For this review, take the finished solid that the model builds, in its own axes (mm). Round coordinates to 2 decimals unless told otherwise and drop trailing zeros. Write each loop counter-clockwise with the first axis right and the second up, starting at its lowest first coordinate (ties: lowest second). Pieces come first, ordered by that corner, then holes. Notation, with made-up numbers: (46, 86.5) -> (51, 86.5) arc R33 ccw to (51, 114.5) -> close; hole circle Ø1 at (71, 6). An arc over 180 degrees is marked (long way). Answer as CSV lines item,"result". Start each with the question number.
Item 1: Take a section at B-B on x = -5.5. Give the boundary of the cut face in (y, z).
Item 2: Wall thickness on probe 1 along Z at (x, y) = (4.5, -0.1); probe 2 along X at (y, z) = (-1.3, 112); probe 3 along Z at (x, y) = (3, -0.9): over which ranges is each line inside the solid? List them lowest first. Write a range as from..to.
Item 3: For pin 1 Ø1.5 at (y, z) = (-1.5, 98.5) entering from +X, flat-tipped, find the tip position at first contact; note if it passes through.
Item 4: Take a section at C-C on z = 44.5. Give the boundary of the cut face in (x, y), then the cut area to 3 significant figures.
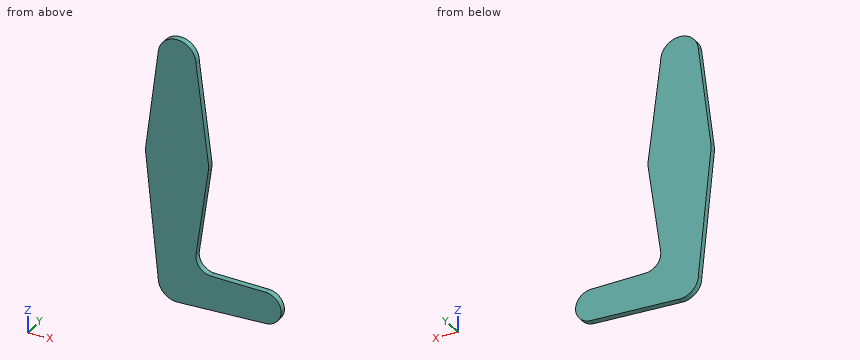
```python
from build123d import *

# Parameters (mm, degrees)
F0_R     = 3.175
F1_DEPTH = 3.048


with BuildPart() as f1:
    # F0 (on Front) → F1 (new body)
    with BuildSketch(Plane.XZ):
        with BuildLine():
            ThreePointArc((9.525, 114.3), (0.596483242, 123.8063048942), (-9.4502929642, 115.490625))
            ThreePointArc((-9.4502929642, 115.490625), (-7.14375, 107.9998046905), (0, 104.775))
            ThreePointArc((0, 104.775), (6.7351920908, 107.5648079092), (9.525, 114.3))
        make_face()
        with BuildLine():
            ThreePointArc((3.175, 114.3), (2.2450640303, 112.0549359697), (0, 111.125))
            ThreePointArc((0, 111.125), (-2.2450640303, 116.5450640303), (3.175, 114.3))
        make_face(mode=Mode.SUBTRACT)
        with BuildLine():
            Line((0, 47.625), (0, 9.525))
            ThreePointArc((0, 9.525), (6.7351920908, 6.7351920908), (9.525, 0))
            Line((9.525, 0), (36.5125, 0))
            ThreePointArc((36.5125, 0), (38.8886909991, 5.663545572), (44.5945783487, 7.9361831727))
            Line((44.5945783487, 7.9361831727), (17.2606145929, 8.4341428668))
            ThreePointArc((17.2606145929, 8.4341428668), (11.3562252192, 11.224257518), (9.5333913565, 17.4951290964))
            Line((9.5333913565, 17.4951290964), (15.7189155447, 61.2793426425))
            ThreePointArc((15.7189155447, 61.2793426425), (10.4106361345, 51.5152480094), (0, 47.625))
        make_face()
        with BuildLine():
            ThreePointArc((-15.7942028036, 61.9003804205), (-10.644756084, 51.722700101), (0, 47.625))
            Line((0, 47.625), (0, 60.325))
            ThreePointArc((0, 60.325), (-3.175, 63.5), (0, 66.675))
            Line((0, 66.675), (0, 79.375))
            ThreePointArc((0, 79.375), (-10.5003255158, 75.40625), (-15.7504882737, 65.484375))
            ThreePointArc((-15.7504882737, 65.484375), (-15.8738192656, 63.6936154008), (-15.7942028036, 61.9003804205))
        make_face()
        with BuildLine():
            Line((0, 100.0252), (0, 79.375))
            ThreePointArc((0, 79.375), (10.4912828548, 75.4142187767), (15.7474569047, 65.5082893304))
            Line((15.7474569047, 65.5082893304), (9.525, 114.3))
            ThreePointArc((9.525, 114.3), (6.7351920908, 107.5648079092), (0, 104.775))
            Line((0, 104.775), (0, 100.0252))
        make_face()
        with BuildLine():
            ThreePointArc((44.5945783487, 7.9361831727), (38.8886909991, 5.663545572), (36.5125, 0))
            ThreePointArc((36.5125, 0), (38.9380895153, -5.7116327839), (44.7324052746, -7.9324746146))
            ThreePointArc((44.7324052746, -7.9324746146), (50.1616327839, -5.5119104847), (52.3875, 0))
            ThreePointArc((52.3875, 0), (50.113545572, 5.5613090009), (44.5945783487, 7.9361831727))
        make_face()
        with BuildLine():
            ThreePointArc((47.625, 0), (44.45, -3.175), (41.275, 0))
            ThreePointArc((41.275, 0), (44.45, 3.175), (47.625, 0))
        make_face(mode=Mode.SUBTRACT)
        with BuildLine():
            Line((-9.4502929642, 115.490625), (-15.7504882737, 65.484375))
            ThreePointArc((-15.7504882737, 65.484375), (-10.5003255158, 75.40625), (0, 79.375))
            Line((0, 79.375), (0, 100.0252))
            Line((0, 100.0252), (0, 104.775))
            ThreePointArc((0, 104.775), (-7.14375, 107.9998046905), (-9.4502929642, 115.490625))
        make_face()
        with Locations((-3.175, 100.0252)):
            Circle(F0_R, mode=Mode.SUBTRACT)
        with BuildLine():
            Line((0, 60.325), (0, 47.625))
            ThreePointArc((0, 47.625), (10.4106361345, 51.5152480094), (15.7189155447, 61.2793426425))
            ThreePointArc((15.7189155447, 61.2793426425), (15.8359308105, 62.3869320038), (15.875, 63.5))
            ThreePointArc((15.875, 63.5), (15.8430821396, 64.5061676396), (15.7474569047, 65.5082893304))
            ThreePointArc((15.7474569047, 65.5082893304), (10.4912828548, 75.4142187767), (0, 79.375))
            Line((0, 79.375), (0, 66.675))
            ThreePointArc((0, 66.675), (2.2450640303, 65.7450640303), (3.175, 63.5))
            ThreePointArc((3.175, 63.5), (2.2450640303, 61.2549359697), (0, 60.325))
        make_face()
        with BuildLine():
            ThreePointArc((3.175, 0), (-2.2450640303, -2.2450640303), (0, 3.175))
            Line((0, 3.175), (0, 9.525))
            ThreePointArc((0, 9.525), (-6.7351920908, 6.7351920908), (-9.525, 0))
            ThreePointArc((-9.525, 0), (-6.7351920908, -6.7351920908), (0, -9.525))
            Line((0, -9.525), (0.6773435479, -9.500885786))
            ThreePointArc((0.6773435479, -9.500885786), (6.9705567315, -6.4912990883), (9.525, 0))
            Line((9.525, 0), (3.175, 0))
        make_face()
        with BuildLine():
            Line((36.5125, 0), (9.525, 0))
            ThreePointArc((9.525, 0), (6.9705567315, -6.4912990883), (0.6773435479, -9.500885786))
            Line((0.6773435479, -9.500885786), (44.7324052746, -7.9324746146))
            ThreePointArc((44.7324052746, -7.9324746146), (38.9380895153, -5.7116327839), (36.5125, 0))
        make_face()
        with BuildLine():
            ThreePointArc((-9.525, 0), (-6.7351920908, 6.7351920908), (0, 9.525))
            Line((0, 9.525), (0, 47.625))
            ThreePointArc((0, 47.625), (-10.644756084, 51.722700101), (-15.7942028036, 61.9003804205))
            Line((-15.7942028036, 61.9003804205), (-9.525, 0))
        make_face()
        with BuildLine():
            Line((0, 9.525), (0, 3.175))
            ThreePointArc((0, 3.175), (2.2450640303, 2.2450640303), (3.175, 0))
            Line((3.175, 0), (9.525, 0))
            ThreePointArc((9.525, 0), (6.7351920908, 6.7351920908), (0, 9.525))
        make_face()
        with BuildLine():
            ThreePointArc((0, -9.525), (0.3388863295, -9.5189695375), (0.6773435479, -9.500885786))
            Line((0.6773435479, -9.500885786), (0, -9.525))
        make_face()
        with BuildLine():
            ThreePointArc((3.175, 114.3), (-2.2450640303, 116.5450640303), (0, 111.125))
            ThreePointArc((0, 111.125), (2.2450640303, 112.0549359697), (3.175, 114.3))
        make_face()
        with BuildLine():
            ThreePointArc((47.625, 0), (44.45, 3.175), (41.275, 0))
            ThreePointArc((41.275, 0), (44.45, -3.175), (47.625, 0))
        make_face()
        with Locations((-3.175, 100.0252)):
            Circle(F0_R)
        with BuildLine():
            ThreePointArc((0, 66.675), (-3.175, 63.5), (0, 60.325))
            Line((0, 60.325), (0, 63.5))
            Line((0, 63.5), (0, 66.675))
        make_face()
        with BuildLine():
            Line((0, 63.5), (0, 60.325))
            ThreePointArc((0, 60.325), (2.2450640303, 61.2549359697), (3.175, 63.5))
            ThreePointArc((3.175, 63.5), (2.2450640303, 65.7450640303), (0, 66.675))
            Line((0, 66.675), (0, 63.5))
        make_face()
        with BuildLine():
            Line((0, 3.175), (0, 0))
            Line((0, 0), (3.175, 0))
            ThreePointArc((3.175, 0), (2.2450640303, 2.2450640303), (0, 3.175))
        make_face()
        with BuildLine():
            Line((3.175, 0), (0, 0))
            Line((0, 0), (0, 3.175))
            ThreePointArc((0, 3.175), (-2.2450640303, -2.2450640303), (3.175, 0))
        make_face()
    extrude(amount=F1_DEPTH)


solid = f1.part
```
Output values:
1,outline,"(-3.05, -7.78) -> (0, -7.78) -> (0, 122.08) -> (-3.05, 122.08) -> close"
2,probe 1,"z = -9.36..122.69"
2,probe 2,"x = -9.89..9.82"
2,probe 3,"z = -9.42..123.34"
3,pin 1,"stops at x = 11.64"
4,outline,"(-14.03, -3.05) -> (13.35, -3.05) -> (13.35, 0) -> (-14.03, 0) -> close"
4,area,"83.5 mm^2"
